Verification items for the finished model (mm, model axes). Coordinates: 2 decimals unless noted, no trailing zeros. Order: outer loops, then holes, each group sorted by start corner. A loop starts at its lowest first (then second) coordinate and runs counter-clockwise, first axis right, second up. Notation, with made-up numbers: (-31.75, 1.25) -> (-10.75, 1.25) arc R17 ccw to (-10.75, 15.25) -> close; hole circle Ø4 at (18, 76). An arc over 180 degrees is marked (long way). Answer as CSV lines item,"result".
```python
from build123d import *

# Parameters (mm, degrees)
F0_W         = 140
F0_H         = 280
F1_DEPTH     = 95
F2_R         = 15
F3_T1_DEPTH  = 140
F3_T4_ANGLE  = 90
F3_T6_ANGLE  = 90
F3_T8_ANGLE  = 90
F3_T10_ANGLE = 90
F3_T12_ANGLE = 90
F3_T14_ANGLE = 90
F3_T16_ANGLE = 90
F3_T18_ANGLE = 90
F4_W         = 110
F4_H         = 120
F5_DEPTH     = 8
F6_R         = 7.99999


# Not quite as in the source:
# - a fillet or chamfer that OpenCascade refuses, or shapes differently, is made with other operations: its cross-section is extruded or revolved along the edge and cut away or added
# - a fillet or chamfer is up to 0.001 mm smaller than in the source, because OpenCascade refuses the exact size


with BuildPart() as f1:
    # F0 (on Top) → F1 (new body)
    with BuildSketch(Plane.XY):
        Rectangle(F0_W, F0_H)
    extrude(amount=F1_DEPTH)

    # F2
    f2_edges = [f1.edges().sort_by_distance(p)[0] for p in [
        (70, -140, 47.5),
        (70, 140, 47.5),
        (70, 0, 0),
        (70, 0, 95),
        (-70, 140, 47.5),
        (-70, -140, 47.5),
        (-70, 0, 0),
        (-70, 0, 95),
    ]]
    fillet(f2_edges, radius=F2_R)

    # F3: fillet of radius 35 on 4 edges, made by hand

    # F3_s2 → F3_t1 (cut)
    with BuildSketch(Plane.YZ.offset(-70)):
        with BuildLine():
            ThreePointArc((-140, 60), (-129.7487373415, 84.7487373415), (-105, 95))
            Line((-105, 95), (-140, 95))
            Line((-140, 95), (-140, 60))
        make_face()
        with BuildLine():
            ThreePointArc((-140, 35), (-129.7487373415, 10.2512626585), (-105, 0))
            Line((-105, 0), (-140, 0))
            Line((-140, 0), (-140, 35))
        make_face()
        with BuildLine():
            ThreePointArc((105, 95), (129.7487373415, 84.7487373415), (140, 60))
            Line((140, 60), (140, 95))
            Line((140, 95), (105, 95))
        make_face()
        with BuildLine():
            ThreePointArc((105, 0), (129.7487373415, 10.2512626585), (140, 35))
            Line((140, 35), (140, 0))
            Line((140, 0), (105, 0))
        make_face()
    extrude(amount=F3_T1_DEPTH, mode=Mode.SUBTRACT)

    # F3_s3 → F3_t4 (revolve, cut)
    with BuildSketch(Plane.XZ.offset(-105)):
        with BuildLine():
            ThreePointArc((70, 15), (65.6066017178, 4.3933982822), (55, 0))
            Line((55, 0), (70, 0))
            Line((70, 0), (70, 15))
        make_face()
    revolve(axis=Axis((70, 105, 35), (1, 0, 0)), revolution_arc=F3_T4_ANGLE, mode=Mode.SUBTRACT)

    # F3_s5 → F3_t6 (revolve, cut)
    with BuildSketch(Plane.XY.offset(35)):
        with BuildLine():
            ThreePointArc((-70, 125), (-65.6066017178, 135.6066017178), (-55, 140))
            Line((-55, 140), (-70, 140))
            Line((-70, 140), (-70, 125))
        make_face()
    revolve(axis=Axis((-70, 105, 35), (-1, 0, 0)), revolution_arc=F3_T6_ANGLE, mode=Mode.SUBTRACT)

    # F3_s7 → F3_t8 (revolve, cut)
    with BuildSketch(Plane.XY.offset(60)):
        with BuildLine():
            ThreePointArc((70, 125), (65.6066017178, 135.6066017178), (55, 140))
            Line((55, 140), (70, 140))
            Line((70, 140), (70, 125))
        make_face()
    revolve(axis=Axis((70, 105, 60), (1, 0, 0)), revolution_arc=F3_T8_ANGLE, mode=Mode.SUBTRACT)

    # F3_s9 → F3_t10 (revolve, cut)
    with BuildSketch(Plane.XZ.offset(-105)):
        with BuildLine():
            ThreePointArc((-70, 80), (-65.6066017178, 90.6066017178), (-55, 95))
            Line((-55, 95), (-70, 95))
            Line((-70, 95), (-70, 80))
        make_face()
    revolve(axis=Axis((-70, 105, 60), (-1, 0, 0)), revolution_arc=F3_T10_ANGLE, mode=Mode.SUBTRACT)

    # F3_s11 → F3_t12 (revolve, cut)
    with BuildSketch(Plane.XZ.offset(105)):
        with BuildLine():
            ThreePointArc((-70, 15), (-65.6066017178, 4.3933982822), (-55, 0))
            Line((-55, 0), (-70, 0))
            Line((-70, 0), (-70, 15))
        make_face()
    revolve(axis=Axis((-70, -105, 35), (-1, 0, 0)), revolution_arc=F3_T12_ANGLE, mode=Mode.SUBTRACT)

    # F3_s13 → F3_t14 (revolve, cut)
    with BuildSketch(Plane.XY.offset(35)):
        with BuildLine():
            ThreePointArc((70, -125), (65.6066017178, -135.6066017178), (55, -140))
            Line((55, -140), (70, -140))
            Line((70, -140), (70, -125))
        make_face()
    revolve(axis=Axis((70, -105, 35), (1, 0, 0)), revolution_arc=F3_T14_ANGLE, mode=Mode.SUBTRACT)

    # F3_s15 → F3_t16 (revolve, cut)
    with BuildSketch(Plane.XY.offset(60)):
        with BuildLine():
            ThreePointArc((-70, -125), (-65.6066017178, -135.6066017178), (-55, -140))
            Line((-55, -140), (-70, -140))
            Line((-70, -140), (-70, -125))
        make_face()
    revolve(axis=Axis((-70, -105, 60), (-1, 0, 0)), revolution_arc=F3_T16_ANGLE, mode=Mode.SUBTRACT)

    # F3_s17 → F3_t18 (revolve, cut)
    with BuildSketch(Plane.XZ.offset(105)):
        with BuildLine():
            ThreePointArc((70, 80), (65.6066017178, 90.6066017178), (55, 95))
            Line((55, 95), (70, 95))
            Line((70, 95), (70, 80))
        make_face()
    revolve(axis=Axis((70, -105, 60), (1, 0, 0)), revolution_arc=F3_T18_ANGLE, mode=Mode.SUBTRACT)

    # F4 (on face) → F5 (join)
    with BuildSketch(Plane.XY.offset(95)):
        with Locations((0, 45)):
            Rectangle(F4_W, F4_H)
    extrude(amount=F5_DEPTH)

    # F6 (radius 8 in the source; OpenCascade refuses exactly that, so slightly less here)
    f6_edges = [f1.edges().sort_by_distance(p)[0] for p in [
        (0, 105, 103),
        (-55, 45, 103),
        (0, -15, 103),
        (55, 45, 103),
    ]]
    fillet(f6_edges, radius=F6_R)


solid = f1.part
```
Item 1: Thickness scan on line 1 (Z direction, x = 28, y = -62); line 2 (Z direction, x = -33, y = 97.5); line 3 (X direction, y = -75, z = 87). Record the ranges inside material, lowest first.
Answer list:
line 1,"0 to 95"
line 2,"0 to 102.98"
line 3,"-68.27 to 68.27"
Item 2: Depth check by flat-ended pin: pin 1 Ø1.5 at (x, y) = (14.5, -11.5) entering from +Z; pin 2 Ø3 at (x, z) = (51.5, 16.5) entering from -Y; pin 3 Ø10 at (x, z) = (-51.5, 78.5) entering from +Y. Enter the tip coordinate at first touch or a pass-through.
Answer list:
pin 1,"z = 102.07"
pin 2,"y = -135.59"
pin 3,"y = 137.29"
Item 3: Section check B-B, the plane y = -31. Record the boundary of the cut face in (x, z).
Answer list:
outline,"(-70, 15) arc R15 ccw to (-55, 0) -> (55, 0) arc R15 ccw to (70, 15) -> (70, 80) arc R15 ccw to (55, 95) -> (-55, 95) arc R15 ccw to (-70, 80) -> close"
